Input: part model. Units: mm. Frame: model coordinates. A direction names the side the tool comes from. Coordinates: 2 decimals unless noted, no trailing zeros. Loops run counter-clockwise (first coordinate to the right, second up) from the corner with the lowest first, then second, coordinate; pieces in that order, holes last. Notation, with made-up numbers: (-22.5, -6) - (6.5, -6) arc R29 cw to (6.5, 26) - close; hole circle Ø10 at (29.5, 31). An arc over 180 degrees is marked (long way). Write item = value, one per line. Start each with the question number.
from build123d import *

# Parameters (mm, degrees)
SKETCH_1_W          = 20
SKETCH_1_H          = 90
EXTRUDE_1_DEPTH     = 4
SKETCH_2_W          = 20
SKETCH_2_H          = 4
EXTRUDE_2_DEPTH     = 20.1
SKETCH_3_W          = 20
SKETCH_3_H          = 4
EXTRUDE_3_DEPTH     = 24.1
SKETCH_4_W          = 20
SKETCH_4_H          = 4
EXTRUDE_4_DEPTH     = 20.1
SKETCH_5_R          = 2.6
CUT_EXTRUDE_1_DEPTH = 20
SKETCH_6_R          = 2.6
CUT_EXTRUDE_2_DEPTH = 20
SKETCH_7_R          = 2.6
CUT_EXTRUDE_3_DEPTH = 20
SKETCH_9_R          = 1.6
CUT_EXTRUDE_4_DEPTH = 20
EXTRUDE_6_DEPTH     = 3
SKETCH_14_W         = 4
SKETCH_14_H         = 20
EXTRUDE_7_DEPTH     = 60
SKETCH_15_W         = 4
SKETCH_15_H         = 20
EXTRUDE_8_DEPTH     = 16
SKETCH_17_R         = 2.6
CUT_EXTRUDE_6_DEPTH = 20


with BuildPart() as part:
    # 草图1 → 凸台-拉伸1 (new body)
    with BuildSketch(Plane.XY):
        with Locations((-19.209677061, -2.260885663)):
            Rectangle(SKETCH_1_W, SKETCH_1_H)
    extrude(amount=EXTRUDE_1_DEPTH)

    # 草图2 → 凸台-拉伸2 (add)
    with BuildSketch(Plane.XY.offset(4)):
        with Locations((-19.209677061, -45.260885663)):
            Rectangle(SKETCH_2_W, SKETCH_2_H)
    extrude(amount=EXTRUDE_2_DEPTH)

    # 草图3 → 凸台-拉伸3 (add)
    with BuildSketch(Plane(origin=(0, -47.260885663, 0), x_dir=(-1, 0, 0), z_dir=(0, -1, 0))):
        with Locations((19.209677061, -22.1)):
            Rectangle(SKETCH_3_W, SKETCH_3_H)
    extrude(amount=EXTRUDE_3_DEPTH)

    # 草图4 → 凸台-拉伸4 (add)
    with BuildSketch(Plane(origin=(0, 0, 20.1), x_dir=(-1, 0, 0), z_dir=(0, 0, -1))):
        with Locations((19.209677061, -69.360885663)):
            Rectangle(SKETCH_4_W, SKETCH_4_H)
    extrude(amount=EXTRUDE_4_DEPTH)

    # 草图5 → 切除-拉伸1 (cut)
    with BuildSketch(Plane(origin=(0, -47.260885663, 0), x_dir=(-1, 0, 0), z_dir=(0, -1, 0))):
        with Locations((19.209677061, -10.094759339)):
            Circle(SKETCH_5_R)
    extrude(amount=-CUT_EXTRUDE_1_DEPTH, mode=Mode.SUBTRACT)

    # 草图6 → 切除-拉伸2 (cut)
    with BuildSketch(Plane(origin=(0, 0, 20.1), x_dir=(-1, 0, 0), z_dir=(0, 0, -1))):
        with Locations((19.209677061, -57.310885663)):
            Circle(SKETCH_6_R)
    extrude(amount=-CUT_EXTRUDE_2_DEPTH, mode=Mode.SUBTRACT)

    # 草图7 → 切除-拉伸3 (cut)
    with BuildSketch(Plane(origin=(0, -67.360885663, 0), x_dir=(1, 0, 0), z_dir=(0, 1, 0))):
        with Locations((-19.209677061, -10.05)):
            Circle(SKETCH_7_R)
    extrude(amount=-CUT_EXTRUDE_3_DEPTH, mode=Mode.SUBTRACT)

    # 草图9 → 切除-拉伸4 (cut)
    with BuildSketch(Plane(origin=(0, 0, 0), x_dir=(-1, 0, 0), z_dir=(0, 0, -1))):
        with Locations((19.209677061, 37.739114337)):
            Circle(SKETCH_9_R)
        with Locations((19.209677061, -38.260885663)):
            Circle(SKETCH_9_R)
    extrude(amount=-CUT_EXTRUDE_4_DEPTH, mode=Mode.SUBTRACT)

    # 草图13 → 凸台-拉伸6 (add)
    with BuildSketch(Plane.ZY.offset(29.209677061)):
        Polygon((4, -11.848280973), (24.1, -43.260885663), (4, -43.260885663), align=None)
    extrude(amount=-EXTRUDE_6_DEPTH)

    # 草图14 → 凸台-拉伸7 (add)
    with BuildSketch(Plane.ZY.offset(29.209677061)):
        with Locations((2, 32.739114337)):
            Rectangle(SKETCH_14_W, SKETCH_14_H)
    extrude(amount=EXTRUDE_7_DEPTH)

    # 草图15 → 凸台-拉伸8 (add)
    with BuildSketch(Plane.XY.offset(4)):
        with Locations((-87.209677061, 32.739114337)):
            Rectangle(SKETCH_15_W, SKETCH_15_H)
    extrude(amount=EXTRUDE_8_DEPTH)

    # 草图17 → 切除-拉伸6 (cut)
    with BuildSketch(Plane.ZY.offset(89.209677061)):
        with Locations((10, 32.739114337)):
            Circle(SKETCH_17_R)
    extrude(amount=-CUT_EXTRUDE_6_DEPTH, mode=Mode.SUBTRACT)


solid = part.part
Item 1: Ray query, line 1 (Y direction, x = -20, z = 18.25); line 2 (Y direction, x = -87.5, z = 10); line 3 (X direction, y = -46.5, z = 11.75). Return the intervals inside material, ascending.
Item 2: Cut plane B-B on y = 26. Return loops of the section in (x, z).
Item 3: Access query for faces 1 (the cylindrical face through (-21.61, -58.31, 22.07)), 2 (the flat face through (-66, 22.739, 3)), 3 (the flat face through (-17, -67.361, 12)), 4 (the flat face through (-85.21, 33, 14)), 5 (the flat face through (-21, 18, 4)). Directions: +Z, -Z, +X, -X, +Y, -Y. A direction counts if a zero-diameter tool reaches every point of the face in a straight line with its end or side. Return the directions, or none.
Item 4: Pin query (flat end, axial travel): pin 1 (6 mm diameter, centred on y = 28, z = 9, fed in from +X); pin 2 (12 mm diameter, centred on x = -24.5, y = 5, fed in from +Z); pin 3 (1.2 mm diameter, centred on x = -87, y = 29.5, fed in from +Z). Return the tip coordinate at first contact, or that it passes through.
Item 5: Cut plane D-D on y = 11. Return loops of the section in (x, z), plus the area to 3 significant figures.
Item 6: Pull-direction query (Z, two-part tool) for faces 6 (the cylindrical face through (-87.24, 30.2, 9.44)), 7 (the flat face through (-17, -71.361, 12)), 8 (the cylindrical face through (-21.807, -69.333, 9.936)), 9 (the flat face through (-22, 17, 0)); classes: pulls with the +Z half, pulls with the -Z half, needs draft (parallel to the pull), parting line crosses it, or undercut.
Item 7: Cut plane A-A on z = 16.75. Return loops of the section in (x, y).
Item 8: Cut plane C-C on x = -82. Return loops of the section in (y, z).
Recorded:
q1.line_1 = -71.36 to -67.36, -47.26 to -43.26
q1.line_2 = 22.74 to 30.14, 35.34 to 42.74
q1.line_3 = -29.21 to -21.21, -17.2 to -9.21
q2.outline = (-89.21, 0) - (-9.21, 0) - (-9.21, 4) - (-85.21, 4) - (-85.21, 20) - (-89.21, 20) - close
q3.face_1 = +Z, -Z
q3.face_2 = +Z, -Z, -X, -Y
q3.face_3 = -Z, +X, -X
q3.face_4 = +Z, +X, +Y, -Y
q3.face_5 = +Z, +X, +Y
q4.pin_1 = -85.21
q4.pin_2 = 4
q4.pin_3 = 20
q5.outline = (-29.21, 0) - (-9.21, 0) - (-9.21, 4) - (-29.21, 4) - close
q5.area = 80.0 mm²
q6.face_6 = undercut
q6.face_7 = needs draft
q6.face_8 = undercut
q6.face_9 = pulls with the -Z half
q7.outline = (-89.21, 22.74) - (-85.21, 22.74) - (-85.21, 42.74) - (-89.21, 42.74) - close; (-29.21, -71.36) - (-9.21, -71.36) - (-9.21, -67.36) - (-29.21, -67.36) - close; (-29.21, -47.26) - (-9.21, -47.26) - (-9.21, -43.26) - (-26.21, -43.26) - (-26.21, -31.77) - (-29.21, -31.77) - close
q8.outline = (22.74, 0) - (42.74, 0) - (42.74, 4) - (22.74, 4) - close
